from build123d import *

# Parameters (mm, degrees)
SKETCH003_R         = 39
PAD002_DEPTH        = 2
PAD009_DEPTH        = 4
SKETCH011_W         = 6
SKETCH011_H         = 13
SKETCH011_R         = 1.5
PAD011_DEPTH        = 10
PAD012_DEPTH        = 2
SKETCH013_R         = 2
SKETCH013_R_2       = 39
POCKET_DEPTH        = 0.001
POCKET_DEPTH_BACK   = 14.001
PAD003_DEPTH        = 29.5
PAD006_DEPTH        = 0.5
LINEARPATTERN_COUNT = 7
LINEARPATTERN_PITCH = 10


with BuildPart() as part:
    # Sketch003 → Pad002 (new body)
    with BuildSketch(Plane.XY):
        with BuildLine():
            Line((-42.5, 35.5), (-42.5, -42.5))
            Line((-42.5, -42.5), (35.5, -42.5))
            ThreePointArc((35.5, -42.5), (40.449747, -40.449747), (42.5, -35.5))
            Line((42.5, -35.5), (42.5, 35.5))
            ThreePointArc((42.5, 35.5), (40.449747, 40.449747), (35.5, 42.5))
            Line((35.5, 42.5), (-35.5, 42.5))
            ThreePointArc((-35.5, 42.5), (-40.449747, 40.449747), (-42.5, 35.5))
        make_face()
        Circle(SKETCH003_R, mode=Mode.SUBTRACT)
    extrude(amount=PAD002_DEPTH)

    # Sketch009 → Pad009 (join)
    with BuildSketch(Plane.XY):
        with BuildLine():
            Line((-42.5, -31), (-42.5, -50))
            ThreePointArc((-42.5, -50), (-41.035534, -53.535534), (-37.5, -55))
            Line((-37.5, -55), (-12.5, -55))
            Line((-12.5, -55), (-12.5, -40))
            Line((-12.5, -40), (-35.5, -40))
            ThreePointArc((-40, -35.5), (-38.681981, -38.681981), (-35.5, -40))
            Line((-40, -31), (-40, -35.5))
            Line((-42.5, -31), (-40, -31))
        make_face()
    extrude(amount=PAD009_DEPTH)

    # Sketch011 → Pad011 (join)
    with BuildSketch(Plane.XY.offset(4)):
        with Locations((-15.5, -48.5)):
            Rectangle(SKETCH011_W, SKETCH011_H)
        with Locations((-15.5, -45.25)):
            Circle(SKETCH011_R, mode=Mode.SUBTRACT)
        with Locations((-15.5, -51.75)):
            Circle(SKETCH011_R, mode=Mode.SUBTRACT)
    extrude(amount=PAD011_DEPTH)

    # Sketch012 → Pad012 (join)
    with BuildSketch(Plane.XY):
        with BuildLine():
            Line((-60, 37.5), (-60, 25.5))
            ThreePointArc((-60, 25.5), (-58.535534, 21.964466), (-55, 20.5))
            Line((-55, 20.5), (-35.5, 20.5))
            Line((-35.5, 20.5), (-35.5, 42.5))
            Line((-35.5, 42.5), (-55, 42.5))
            ThreePointArc((-55, 42.5), (-58.535534, 41.035534), (-60, 37.5))
        make_face()
    extrude(amount=PAD012_DEPTH)

    # Sketch013 → Pocket (cut, two sides)
    with BuildSketch(Plane.XY) as pocket_sk:
        with Locations((-35.5, 35.5)):
            Circle(SKETCH013_R)
        with Locations((35.5, 35.5)):
            Circle(SKETCH013_R)
        with Locations((35.5, -35.5)):
            Circle(SKETCH013_R)
        with Locations((-35.5, -35.5)):
            Circle(SKETCH013_R)
        Circle(SKETCH013_R_2)
    extrude(amount=-POCKET_DEPTH, mode=Mode.SUBTRACT)
    extrude(pocket_sk.sketch, amount=POCKET_DEPTH_BACK, mode=Mode.SUBTRACT)

    # Sketch002 → Pad003 (join, symmetric)
    with BuildSketch(Plane.XZ):
        Polygon((22.5, 11.326153), (42.5, 2), (42.5, 0.8), (22.5, 10.126153), align=None)
    extrude(amount=PAD003_DEPTH, both=True)

    # Sketch006 → Pad006 (join, symmetric)
    with BuildSketch(Plane.XZ.offset(-30)):
        Polygon((22.5, 11.326153), (42.5, 2), (42.5, 0), (22.5, 0), align=None)
    pad006 = extrude(amount=PAD006_DEPTH, both=True)

    # LinearPattern: Pad006 ×7
    with Locations(*[(0, -i * LINEARPATTERN_PITCH, 0) for i in range(1, LINEARPATTERN_COUNT)]):
        add(pad006)


with BuildPart() as part_1:
    # Body001 placement: moved
    add(part.part.moved(Location((0, 0, 2))))


solid = part_1.part
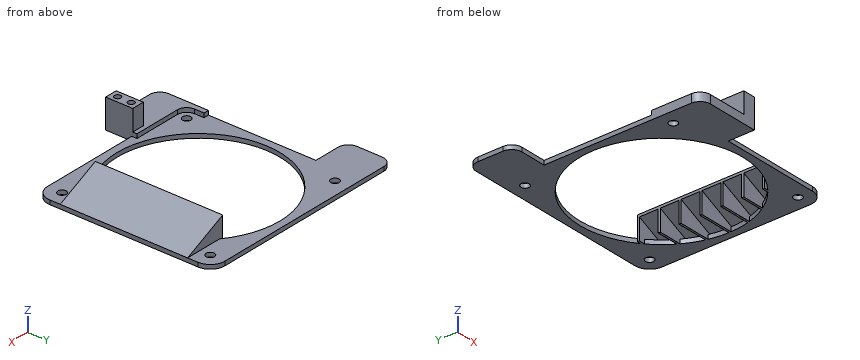
Can you work these out from the model? Positions are in its coordinate system, mm. Give positions to 0.01 mm unless a question says otherwise; leave off trailing zeros. Loops run counter-clockwise (first coordinate to the right, second up) from the corner with the lowest first, then second, coordinate; pieces in that order, holes last. Notation, with made-up numbers: (-19.75, 53.25) -> (38.25, 53.25) arc R34 cw to (38.25, 84.25) -> close; hole circle Ø5 at (11.25, 78.5). An arc over 180 degrees is marked (long way). Write item = value, one per line.
1) Suppose I cut it at A-A on z = 8.25. Give the number of separate pieces and of enclosed holes in the cut face, then the cut area to 3 significant figures.
Check result:
separate_pieces = 2
enclosed_holes = 2
area = 279 mm2
2) Suppose I cut it at C-C on y = -7.5. Write out the boundary of the cut face in (x, z).
Check result:
outline = (-42.5, 2) -> (-38.27, 2) -> (-38.27, 4) -> (-42.5, 4) -> close; (22.5, 12.13) -> (39.93, 4) -> (38.27, 4) -> (38.27, 2) -> (42.5, 2) -> (42.5, 4) -> (22.5, 13.33) -> close
3) Suppose I cut it at B-B on x = 0. Write out the boundary of the cut face in (y, z).
Check result:
outline = (-42.5, 2) -> (-39, 2) -> (-39, 4) -> (-42.5, 4) -> close; (39, 2) -> (42.5, 2) -> (42.5, 4) -> (39, 4) -> close
4) Suppose I cut it at D-D on y = -45.25. Write out the boundary of the cut face in (x, z), then the cut area to 3 significant figures.
Check result:
outline = (-42.5, 2) -> (-12.5, 2) -> (-12.5, 16) -> (-14, 16) -> (-14, 6) -> (-17, 6) -> (-17, 16) -> (-18.5, 16) -> (-18.5, 6) -> (-42.5, 6) -> close
area = 150 mm2
5) I need wall thicknesses on L1, parallel to Y at x = -15.5, z = 11.5; L2, parallel to X at y = -35.5, z = 3.1; L3, parallel to Y at x = -27, z = 5. Which ranges of each line are inside material? Lowest first, please. Write a range as from..to.
Check result:
L1 = -55..-53.25, -50.25..-46.75, -43.75..-42
L2 = -42.5..-37.5, -33.5..-16.15, 16.15..33.5, 37.5..42.5
L3 = -55..-40
6) Will these pins go through, and if not, where does the flat tip stop? pin 1 (5 mm diameter, centred on x = -46.5, y = 27.5, fed in from +Z); pin 2 (3 mm diameter, centred on x = 35.5, y = -17, fed in from +Z); pin 3 (1.6 mm diameter, centred on x = 20, z = 3.5, fed in from -Y).
Check result:
pin_1 = 4
pin_2 = 7.96
pin_3 = -42.5
